```python
from build123d import *

# Parameters (mm, degrees)
SKETCH1_R             = 3
BOSS_EXTRUDE1_DEPTH   = 52.5
CHAMFER1_SIZE         = 0.5
CHAMFER1_SIZE2        = 0.866025404
CHAMFER1_PART_2_SIZE  = 0.5
CHAMFER1_PART_2_SIZE2 = 0.866025404


with BuildPart() as part:
    # Sketch1 → Boss-Extrude1 (new body, symmetric)
    with BuildSketch(Plane(origin=(0, 0, 0), x_dir=(0, 0, -1), z_dir=(1, 0, 0))):
        Circle(SKETCH1_R)
    extrude(amount=BOSS_EXTRUDE1_DEPTH, both=True)

    # Chamfer1
    chamfer1_edges = [part.edges().sort_by_distance(p)[0] for p in [
        (-52.5, 0, 3),
    ]]
    chamfer1_side = [part.faces().sort_by_distance(p)[0] for p in [
        (-52.5, 0, 0),
    ]]
    chamfer(chamfer1_edges, length=CHAMFER1_SIZE, length2=CHAMFER1_SIZE2, reference=chamfer1_side[0])

    # Chamfer1 part 2
    chamfer1_part_2_edges = [part.edges().sort_by_distance(p)[0] for p in [
        (52.5, 0, 3),
    ]]
    chamfer1_part_2_side = [part.faces().sort_by_distance(p)[0] for p in [
        (0, 0, 3),
    ]]
    chamfer(chamfer1_part_2_edges, length=CHAMFER1_PART_2_SIZE, length2=CHAMFER1_PART_2_SIZE2, reference=chamfer1_part_2_side[0])


solid = part.part
```
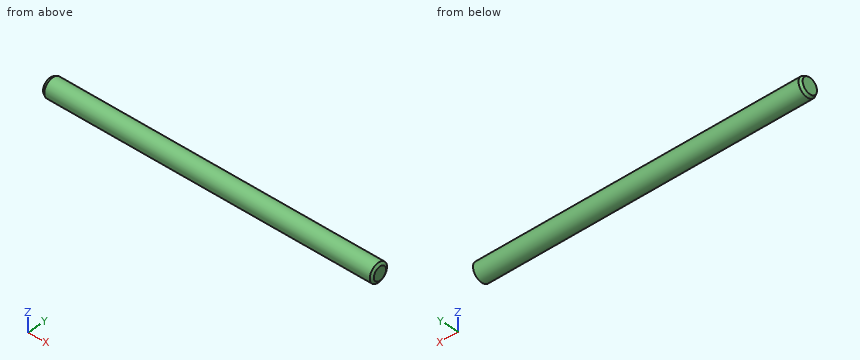
The model under review builds one solid part; all positions refer to its coordinate system, in mm. Give positions to 0.01 mm unless a question says otherwise; leave off trailing zeros. Write each loop counter-clockwise with the first axis right and the second up, starting at its lowest first coordinate (ties: lowest second). Pieces come first, ordered by that corner, then holes. Notation, with made-up numbers: M 0,-35 L 47,-35 A17 cw 47,-26 Z; hole C 61.25,68.5 d1. An arc over 180 degrees is marked long. Write item = value, one per line. Start each with the question number.
Q1. We need section A-A (x = -24). State the section outline as (y, z) points.
Q2. Clearance check with a flat-ended pin moving along its axis: pin 1 (3 mm diameter, centred on x = -1.5, y = -2, fed in from +Z). State where the tip first meets the part, or that it passes through.
Q3. For line 1 (Y direction, x = -44, z = 0.2); line 2 (Y direction, x = 17.5, z = 2.1), list the stretches that pass through material, from the lowest coordinate up.
Result set:
q1.outline = C 0,0 d6
q2.pin_1 = 2.96
q3.line_1 = -2.99 to 2.99
q3.line_2 = -2.14 to 2.14
